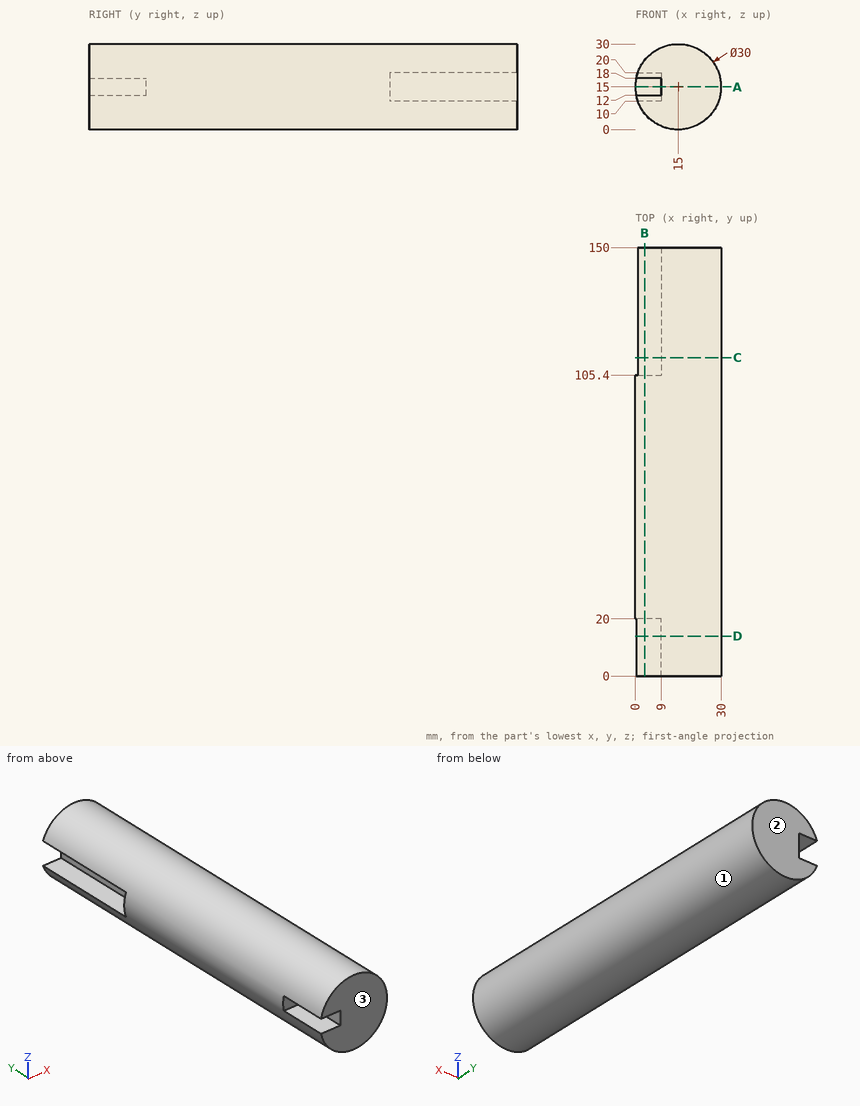
Answer from the drawing. Dimensions are ordinates in mm from the lowest x, y and z of the part. Give positions to 0.01 mm unless a question says otherwise; leave off trailing zeros. Write each loop counter-clockwise with the first axis right and the second up, starting at its lowest first coordinate (ties: lowest second). Pieces come first, ordered by that corner, then holes.
1) For a pull along Y with two mould halves and no side action, classify the marked faces 1, 2 and 3 as pulls with the +Y half, pulls with the -Y half, needs draft (parallel to the pull), parting line crosses it, or undercut.
2) Section A-A (z = 15) is taken. Write down the section's boundary in (x, y).
3) Section B-B (x = 3.25) is taken. Write down the section's boundary in (y, z).
4) Section C-C (y = 111.5) is taken. Write down the section's boundary in (x, z), and give its area (3 significant figures).
5) Given P1, Ø3, axis at y = 129.5, z = 15.5, coming from the -X side; P2, Ø4.5, axis at x = 5, y = 11, coming from the +Z side; P3, Ø4.5, axis at x = 2.5, z = 12.5, coming from the +Y side, each flat-ended and moving along its own axis, determine where each tip first touches the part or whether it passes through.
6) Find the intervals of material crossed by L1, parallel to Y at x = 5, z = 13.5; L2, parallel to Y at x = 6, z = 19.5; L3, parallel to X at y = 63, z = 15.75, in increasing order.
7) Section D-D (y = 14) is taken. Write down the section's boundary in (x, z), and give its area (3 significant figures).
Response:
1. face 1: needs draft
1. face 2: pulls with the +Y half
1. face 3: pulls with the -Y half
2. outline: (0, 20) - (9, 20) - (9, 0) - (30, 0) - (30, 150) - (9, 150) - (9, 105.4) - (0, 105.4) - close
3. outline: (0, 5.68) - (150, 5.68) - (150, 10) - (105.4, 10) - (105.4, 20) - (150, 20) - (150, 24.32) - (0, 24.32) - (0, 18) - (20, 18) - (20, 12) - (0, 12) - close
4. outline: (0.86, 10) arc R15 ccw (long way) to (0.86, 20) - (9, 20) - (9, 10) - close
4. area: 620 mm2
5. P1: stops at x = 9
5. P2: stops at z = 27.84
5. P3: stops at y = 105.4
6. L1: y = 20 to 105.4
6. L2: y = 0 to 105.4
6. L3: x = 0.02 to 29.98
7. outline: (0.3, 12) arc R15 ccw (long way) to (0.3, 18) - (9, 18) - (9, 12) - close
7. area: 653 mm2
